Geometry: final body of the model. Coordinates: model frame, mm. A direction names the side the tool comes from. Round coordinates to 2 decimals unless told otherwise and drop trailing zeros. Loops run counter-clockwise (first coordinate to the right, second up) from the corner with the lowest first, then second, coordinate; pieces in that order, holes last. Notation, with made-up numbers: (-19.75, -26.5) - (0.25, -26.5) arc R8 ccw to (0.25, -11.5) - close; hole circle Ø10 at (-20.5, 81.5). An arc over 180 degrees is marked (long way). Answer as a JSON object with one key per item and string values. Group by question number.
Item 1: First-contact query: pin 1 (2 mm diameter, centred on x = -1, z = -1, fed in from -Y). Flat tip, straight axial feed; report the tip coordinate or a pass-through.
Item 2: Line query: line 1 (Y direction, x = 0, z = -3.5); line 2 (X direction, y = -2, z = 4.75); line 3 (X direction, y = -2.25, z = 2.25). Output: solid intervals per line, ascending.
Item 3: Section C-C (z = -2.25). Return the cut outline in (x, y).
Item 4: Section A-A (y = -1.25). Return the cut outline in (x, z), plus the area to 3 significant figures.
Item 5: Section D-D (z = 2.54). Return the cut outline in (x, y), plus the area to 3 significant figures.
Item 6: Draft query along X for faces 3 (the face through (-3.75, 5, 0)), 4 (the face through (0, 5, 6.25)), 5 (the face through (3.017, -1.726, 4.93)). Return one class per face: released by +X, released by -X, zero draft, split by the parting line, or undercut.
Item 7: Section B-B (x = 2.54). Return the cut outline in (y, z).
Item 8: Reachability of faces 1 (the face through (-2.5, -3.5, 2.5)), 2 (the face through (0, 0, 0)) from +Z, -Z, +X, -X, +Y, -Y: full face, straight path, thin tool, end or side. Return the list, or none.
Autodesk Inventor part; units mm, degrees
ref_plane "YZ Plane" through (0, 0, 0) normal (1, 0, 0) x (0, 1, 0)
ref_plane "XZ Plane" through (0, 0, 0) normal (0, 1, 0) x (-1, 0, 0)
ref_plane "XY Plane" through (0, 0, 0) normal (0, 0, 1) x (1, 0, 0)
sketch "Sketch1" plane through (0, 0, 0) normal (0, 1, 0) x (-1, 0, 0)
  line L0 (3.75, 6.25) -> (-3.75, 6.25)
  line L1 (-3.75, 6.25) -> (-3.75, -6.25)
  line L2 (-3.75, -6.25) -> (3.75, -6.25)
  line L3 (3.75, -6.25) -> (3.75, 6.25)
  point P0 (0, 0)
  dimension "d0" = 7.5
  dimension "d1" = 3.75
  dimension "d2" = 12.5
  dimension "d3" = 6.25
extrude "Extrusion1" add sketch "Sketch1" along normal blind 10
fillet "Fillet1" radius 0.5 8 edges at (3.75, 5, -6.25) (3.75, 5, 6.25) (-3.75, 5, 6.25) (0, 10, 6.25) (3.75, 10, 0) (0, 10, -6.25) (-3.75, 10, 0) (-3.75, 5, -6.25)
sketch "Sketch2" plane through (0, 0, 0) normal (0, -1, 0) x (1, 0, 0)
  circle A0 centre (2.54, 5.08) radius 0.5
  line L0 (3.75, 5.75) -> (3.75, -5.75)
  line L1 (3.75, 1.9877) -> (3.75, 0.9043)
  line L2 (1.2566, 6.25) -> (0.5094, 6.25)
  line L3 (-3.25, 6.25) -> (3.25, 6.25)
  circle A1 centre (2.54, 2.54) radius 0.5
  circle A2 centre (2.54, 0) radius 0.5
  circle A3 centre (2.54, -2.54) radius 0.5
  circle A4 centre (2.54, -5.08) radius 0.5
  circle A5 centre (-2.54, 5.08) radius 0.5
  circle A6 centre (-2.54, 2.54) radius 0.5
  circle A7 centre (-2.54, 0) radius 0.5
  circle A8 centre (-2.54, -2.54) radius 0.5
  circle A9 centre (-2.54, -5.08) radius 0.5
  point P0 (0, 0)
  dimension "d7" = 1
  dimension "d8" = 2.54
  dimension "d9" = 5.08
  dimension "d12" = 2.54
  dimension "d15" = 5.08
extrude "Extrusion2" add sketch "Sketch2" along normal blind 3.5 contours A0 | A1 | A4 | A5 | A6 | A9
properties part number "G5V-1-DC5_Relay"
Values:
{
 "1": {"pin 1": "stops at y = 0"},
 "2": {"line 1": "y = 0 to 10", "line 2": "x = -2.92 to -2.16, 2.16 to 2.92", "line 3": "x = -2.95 to -2.13, 2.13 to 2.95"},
 "3": {"outline": "(-3.75, 0) - (3.75, 0) - (3.75, 9.5) arc R0.5 ccw to (3.25, 10) - (-3.25, 10) arc R0.5 ccw to (-3.75, 9.5) - close"},
 "4": {"outline": "circle Ø1 at (-2.54, -5.08); circle Ø1 at (-2.54, 2.54); circle Ø1 at (-2.54, 5.08); circle Ø1 at (2.54, -5.08); circle Ø1 at (2.54, 2.54); circle Ø1 at (2.54, 5.08)", "area": "4.71 mm^2"},
 "5": {"outline": "(-3.75, 0) - (-3.04, 0) - (-3.04, -3.5) - (-2.04, -3.5) - (-2.04, 0) - (2.04, 0) - (2.04, -3.5) - (3.04, -3.5) - (3.04, 0) - (3.75, 0) - (3.75, 9.5) arc R0.5 ccw to (3.25, 10) - (-3.25, 10) arc R0.5 ccw to (-3.75, 9.5) - close", "area": "81.9 mm^2"},
 "6": {"face 3": "released by -X", "face 4": "zero draft", "face 5": "undercut"},
 "7": {"outline": "(-3.5, -5.58) - (0, -5.58) - (0, -6.25) - (9.5, -6.25) arc R0.5 ccw to (10, -5.75) - (10, 5.75) arc R0.5 ccw to (9.5, 6.25) - (0, 6.25) - (0, 5.58) - (-3.5, 5.58) - (-3.5, 4.58) - (0, 4.58) - (0, 3.04) - (-3.5, 3.04) - (-3.5, 2.04) - (0, 2.04) - (0, -4.58) - (-3.5, -4.58) - close"},
 "8": {"face 1": "+Z, -Z, +X, -X, -Y", "face 2": "-Y"}
}
